Source: CAD feature listing. Evaluate the final solid. Frame: model axes, mm. Face numbers are marked on the shaded views. A direction names the side the tool comes from. Give positions to 0.01 mm unless a question says otherwise; leave off trailing zeros. Order: outer loops, then holes, each group sorted by start corner. A loop starts at its lowest first (then second) coordinate and runs counter-clockwise, first axis right, second up. Notation, with made-up numbers: (-37.75, 89) - (-3.75, 89) arc R22 ccw to (-3.75, 126) - close; hole circle Ø9 at (8, 22.25). An arc over 180 degrees is marked (long way). Write each question's results on one line, items separated by ' | '. Start each with the question number.
Item 1: Contact query for flat-ended pins moving along their axis: pin 1 Ø3 at (x, y) = (4, 16.5) entering from +Z; pin 2 Ø1 at (x, y) = (-1, 12.5) entering from +Z; pin 3 Ø0.6 at (x, y) = (63, 26) entering from +Z. Output: stop coordinate, or through.
Item 2: Line query: line 1 along X through (y, z) = (8.5, 2.25); line 2 along X through (y, z) = (13.5, 3.25); line 3 along Y through (x, z) = (55.5, 1.5). Output: solid intervals per line, ascending.
Item 3: Mould query, pull axis X, two halves, no side actions, for the marked faces 3, 4 and 5. Classes: released by +X, released by -X, zero draft, split by the parting line, or undercut.
Item 4: Set-up query: the marked faces 1 and 2. Return all of +Z, -Z, +X, -X, +Y, -Y with unobstructed straight access to the full face (end or side cutting, diameter ignored); none if empty.
Item 5: Section A-A on z = 4.25. Output: boundary loops of the cut face in (x, y).
Item 6: Section C-C on x = 30.5. Output: boundary loops of the cut face in (y, z), and give its area (3 significant figures).
Item 7: Section D-D on y = 6.25. Output: boundary loops of the cut face in (x, z).
Item 8: Section B-B on y = 11.25. Output: boundary loops of the cut face in (x, z).
```python
from build123d import *

# Parameters (mm, degrees)
F0_W     = 5
F0_H     = 16.8
F0_W_2   = 10
F0_H_2   = 8.8
F0_W_3   = 15.8
F0_H_3   = 8
F1_DEPTH = 1
F0_H_4   = 2
F2_DEPTH = 2.5
F3_DEPTH = 5
F4_DEPTH = 8
F0_W_4   = 2
F5_DEPTH = 6


with BuildPart() as f1:
    # F0 (on Top) → F1 (new body)
    with BuildSketch(Plane.XY):
        Polygon((69, 24.8), (53.2, 24.8), (53.2, 20.8), (53.2, 16.8), (69, 16.8), align=None)
        Polygon((0, 24.8), (0, 20.8), (6, 20.8), (6, 4), (0, 4), (0, 0), (53.2, 0), (53.2, 8), (53.2, 12.4), (48, 12.4), (48, 20.8), (53.2, 20.8), (53.2, 24.8), align=None)
        with Locations((14.5, 12.4)):
            Rectangle(F0_W, F0_H, mode=Mode.SUBTRACT)
        with Locations((36.3, 12.4)):
            Rectangle(F0_W_2, F0_H_2, mode=Mode.SUBTRACT)
        with Locations((61.1, 4)):
            Rectangle(F0_W_3, F0_H_3)
    extrude(amount=F1_DEPTH)

    # F0 (on Top) → F2 (join)
    with BuildSketch(Plane.XY):
        with Locations((61.1, 25.8)):
            Rectangle(F0_W_3, F0_H_4)
        Polygon((69, 8), (69, 16.8), (53.2, 16.8), (53.2, 12.4), (53.2, 8), align=None)
        with Locations((61.1, -1)):
            Rectangle(F0_W_3, F0_H_4)
    extrude(amount=F2_DEPTH)

    # F0 (on Top) → F3 (join)
    with BuildSketch(Plane.XY):
        Polygon((6, 20.8), (0, 20.8), (0, 16.4), (0, 8.4), (0, 4), (6, 4), align=None)
        with Locations((14.5, 12.4)):
            Rectangle(F0_W, F0_H)
        with Locations((36.3, 12.4)):
            Rectangle(F0_W_2, F0_H_2)
        Polygon((53.2, 16.8), (53.2, 20.8), (48, 20.8), (48, 12.4), (53.2, 12.4), align=None)
    extrude(amount=F3_DEPTH)

    # F0 (on Top) → F4 (join)
    with BuildSketch(Plane.XY):
        Polygon((0, 16.4), (0, 20.8), (0, 24.8), (53.2, 24.8), (53.2, 26.8), (-2, 26.8), (-2, 16.4), align=None)
        Polygon((69, 26.8), (69, 24.8), (69, 16.8), (69, 8), (69, 0), (69, -2), (71, -2), (71, 26.8), align=None)
        Polygon((0, 4), (0, 8.4), (-2, 8.4), (-2, -2), (53.2, -2), (53.2, 0), (0, 0), align=None)
    extrude(amount=F4_DEPTH)

    # F0 (on Top) → F5 (join)
    with BuildSketch(Plane.XY):
        with Locations((-1, 12.4)):
            Rectangle(F0_W_4, F0_H_3)
    extrude(amount=F5_DEPTH)


solid = f1.part
```
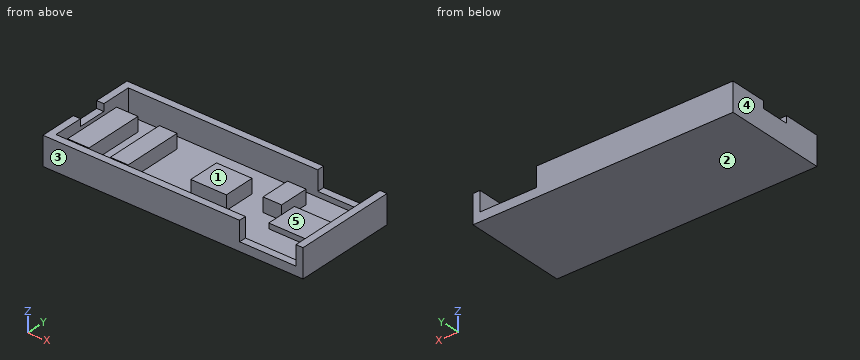
Evaluation:
1) pin 1: stops at z = 5 | pin 2: stops at z = 6 | pin 3: stops at z = 2.5
2) line 1: x = -2 to 6, 12 to 17, 31.3 to 41.3, 53.2 to 71 | line 2: x = -2 to 6, 12 to 17, 31.3 to 41.3, 48 to 53.2, 69 to 71 | line 3: y = -2 to 0, 8 to 16.8, 24.8 to 26.8
3) face 3: zero draft | face 4: released by -X | face 5: undercut
4) face 1: +Z | face 2: -Z, +X, -X, +Y, -Y
5) outline: (-2, -2) - (53.2, -2) - (53.2, 0) - (0, 0) - (0, 4) - (6, 4) - (6, 20.8) - (0, 20.8) - (0, 24.8) - (53.2, 24.8) - (53.2, 26.8) - (-2, 26.8) - close; (12, 4) - (17, 4) - (17, 20.8) - (12, 20.8) - close; (31.3, 8) - (41.3, 8) - (41.3, 16.8) - (31.3, 16.8) - close; (48, 12.4) - (53.2, 12.4) - (53.2, 20.8) - (48, 20.8) - close; (69, -2) - (71, -2) - (71, 26.8) - (69, 26.8) - close
6) outline: (-2, 0) - (26.8, 0) - (26.8, 8) - (24.8, 8) - (24.8, 1) - (0, 1) - (0, 8) - (-2, 8) - close | area: 56.8 mm^2
7) outline: (-2, 0) - (71, 0) - (71, 8) - (69, 8) - (69, 1) - (17, 1) - (17, 5) - (12, 5) - (12, 1) - (6, 1) - (6, 5) - (0, 5) - (0, 8) - (-2, 8) - close
8) outline: (-2, 0) - (71, 0) - (71, 8) - (69, 8) - (69, 2.5) - (53.2, 2.5) - (53.2, 1) - (41.3, 1) - (41.3, 5) - (31.3, 5) - (31.3, 1) - (17, 1) - (17, 5) - (12, 5) - (12, 1) - (6, 1) - (6, 5) - (0, 5) - (0, 6) - (-2, 6) - close
